```python
from build123d import *

# Parameters (mm, degrees)
SKETCH_1_W          = 48.45
SKETCH_1_H          = 34.2
SKETCH_1_W_2        = 28.45
SKETCH_1_H_2        = 14.2
EXTRUDE_1_DEPTH     = 12.25
SKETCH_2_R          = 1.91
CUT_EXTRUDE_1_DEPTH = 33.083066016
SKETCH_4_W          = 13
SKETCH_4_H          = 13.91
EXTRUDE_1_2_DEPTH   = 74.82
SKETCH_5_W          = 13.91
SKETCH_5_H          = 16.23
EXTRUDE_2_DEPTH     = 16
SKETCH_7_R          = 25.25
SKETCH_7_R_2        = 15.25
EXTRUDE_2_2_DEPTH   = 16.23
SKETCH_15_R         = 1.91
CUT_EXTRUDE_6_DEPTH = 97.964478439
SKETCH_16_W         = 13.91
SKETCH_16_H         = 16.23
EXTRUDE_4_DEPTH     = 10
SKETCH_17_R         = 1.91
CUT_EXTRUDE_7_DEPTH = 102.16913771
SKETCH_18_W         = 48.429544624
SKETCH_18_H         = 6.125
CUT_EXTRUDE_8_DEPTH = 105.840616652
SKETCH_19_W         = 34.2
SKETCH_19_H         = 6.125
CUT_EXTRUDE_9_DEPTH = 10


with BuildPart() as part:
    # 草圖1 → Extrude 1 (new body)
    with BuildSketch(Plane(origin=(0, 0, 0), x_dir=(1, 0, 0), z_dir=(0, 1, 0))):
        Rectangle(SKETCH_1_W, SKETCH_1_H)
        Rectangle(SKETCH_1_W_2, SKETCH_1_H_2, mode=Mode.SUBTRACT)
    extrude(amount=EXTRUDE_1_DEPTH)

    # 草圖2 → 除料-伸長1 (cut, through all)
    with BuildSketch(Plane(origin=(0, 12.25, 0), x_dir=(1, 0, 0), z_dir=(0, 1, 0))):
        with Locations(Location((-19.225, 0, 0), (0, 0, 270))):
            Circle(SKETCH_2_R)
        with Locations(Location((19.225, 0, 0), (0, 0, 270))):
            Circle(SKETCH_2_R)
    extrude(amount=-CUT_EXTRUDE_1_DEPTH, mode=Mode.SUBTRACT)

    # 草圖4 → Extrude 1 2 (add)
    with BuildSketch(Plane.XZ):
        with Locations((17.725, 0)):
            Rectangle(SKETCH_4_W, SKETCH_4_H)
    extrude(amount=EXTRUDE_1_2_DEPTH)

    # 草圖5 → Extrude 2 (add)
    with BuildSketch(Plane.ZY.offset(-11.225)):
        with Locations((0, -66.705)):
            Rectangle(SKETCH_5_W, SKETCH_5_H)
    extrude(amount=EXTRUDE_2_DEPTH)

    # 草圖7 → Extrude 2 2 (add)
    with BuildSketch(Plane(origin=(3.626674765, -74.82, 0), x_dir=(1, 0, 0), z_dir=(0, -1, 0))):
        with Locations((-30.978154344, 0)):
            Circle(SKETCH_7_R)
        with Locations((-30.978154344, 0)):
            Circle(SKETCH_7_R_2, mode=Mode.SUBTRACT)
    extrude(amount=-EXTRUDE_2_2_DEPTH)

    # 草圖15 → 除料-伸長6 (cut, through all)
    with BuildSketch(Plane(origin=(0, 0, -6.955), x_dir=(-1, 0, 0), z_dir=(0, 0, -1))):
        with Locations((-4.073383248, -66.705)):
            Circle(SKETCH_15_R)
    extrude(amount=-CUT_EXTRUDE_6_DEPTH, mode=Mode.SUBTRACT)

    # 草圖16 → 填料-伸長4 (add)
    with BuildSketch(Plane(origin=(-60, 0, 0), x_dir=(0, 0, -1), z_dir=(1, 0, 0))):
        with Locations((0, -66.705)):
            Rectangle(SKETCH_16_W, SKETCH_16_H)
    extrude(amount=EXTRUDE_4_DEPTH)

    # 草圖17 → 除料-伸長7 (cut, through all)
    with BuildSketch(Plane(origin=(0, 0, -6.955), x_dir=(-1, 0, 0), z_dir=(0, 0, -1))):
        with Locations((55.812362827, -66.705)):
            Circle(SKETCH_17_R)
    extrude(amount=-CUT_EXTRUDE_7_DEPTH, mode=Mode.SUBTRACT)

    # 草圖18 → 除料-伸長8 (cut, through all)
    with BuildSketch(Plane(origin=(0, 0, -17.1), x_dir=(-1, 0, 0), z_dir=(0, 0, -1))):
        with Locations((0.010227688, 9.1875)):
            Rectangle(SKETCH_18_W, SKETCH_18_H)
    extrude(amount=-CUT_EXTRUDE_8_DEPTH, mode=Mode.SUBTRACT)

    # 草圖19 → 除料-伸長9 (cut)
    with BuildSketch(Plane.ZY.offset(-24.204544624)):
        with Locations((0, 9.1875)):
            Rectangle(SKETCH_19_W, SKETCH_19_H)
    extrude(amount=-CUT_EXTRUDE_9_DEPTH, mode=Mode.SUBTRACT)


solid = part.part
```
Read the model definition and answer for the solid it produces. Units are mm, in the model's axes. A direction names the side the tool comes from. Give positions to 0.01 mm unless a question says otherwise; leave off trailing zeros. Write each loop counter-clockwise with the first axis right and the second up, starting at its lowest first coordinate (ties: lowest second). Pieces come first, ordered by that corner, then holes. Notation, with made-up numbers: (45, -30) -> (69, -30) arc R20 ccw to (69, 7) -> close; hole circle Ø2 at (64, -31.75). An arc over 180 degrees is marked (long way). Answer as a JSON object with one key per item and string values.
1) Section B-B on y = -61.5 is taken. Write down the section's boundary in (x, z) (3 decimals).
Findings below:
{"outline": "(-60, -6.955) -> (-51.625, -6.955) arc R25.25 ccw to (-3.078, -6.955) -> (24.225, -6.955) -> (24.225, 6.955) -> (-3.078, 6.955) arc R25.25 ccw to (-51.625, 6.955) -> (-60, 6.955) -> close; hole circle Ø30.5 at (-27.351, 0)"}
2) Straight lines are drawn through the part: probe 1 along X at (y, z) = (2, 0) (3 decimals); probe 2 along Y at (x, z) = (-13, 12) (3 decimals); probe 3 along Z at (x, y) = (-26.5, -60). For each, find the intervals that lie inside material, in ascending order. Write a range as from..to.
Findings below:
{"probe 1": "x = -24.225..-21.135, -17.315..-14.225, 14.225..17.315, 21.135..24.225", "probe 2": "y = -74.82..-58.59, 0..6.125", "probe 3": "z = -25.24..-15.23, 15.23..25.24"}
3) Section A-A on z = 0 is taken. Write down the section's boundary in (x, y) (3 decimals).
Findings below:
{"outline": "(-60, -74.82) -> (-42.601, -74.82) -> (-42.601, -58.59) -> (-60, -58.59) -> close; (-24.225, 0) -> (-21.135, 0) -> (-21.135, 6.125) -> (-24.225, 6.125) -> close; (-17.315, 0) -> (-14.225, 0) -> (-14.225, 6.125) -> (-17.315, 6.125) -> close; (-12.101, -74.82) -> (24.225, -74.82) -> (24.225, 6.125) -> (21.135, 6.125) -> (21.135, 0) -> (17.315, 0) -> (17.315, 6.125) -> (14.225, 6.125) -> (14.225, 0) -> (11.225, 0) -> (11.225, -58.59) -> (-12.101, -58.59) -> close; hole circle Ø3.82 at (-55.812, -66.705); hole circle Ø3.82 at (4.073, -66.705)"}
4) Flat-ended cylindrical pins translate along their axes: pin 1 Ø3.5 at (x, y) = (-55.81, -66.7) entering from -Z; pin 2 Ø1.8 at (x, y) = (-12, 3.5) entering from +Z; pin 3 Ø3 at (x, y) = (10.5, -53) entering from -Z (3 decimals); pin 4 Ø3 at (y, z) = (-64.5, -17) entering from +X. Find the tip coordinate at first contact, or state that the pin passes through.
Findings below:
{"pin 1": "passes through", "pin 2": "stops at z = 17.1", "pin 3": "stops at z = -6.955", "pin 4": "stops at x = -7.42"}
5) Section C-C on x = -34 is taken. Write down the section's boundary in (y, z), then the cut area to 3 significant figures.
Findings below:
{"outline": "(-74.82, -24.36) -> (-58.59, -24.36) -> (-58.59, -13.72) -> (-74.82, -13.72) -> close; (-74.82, 13.72) -> (-58.59, 13.72) -> (-58.59, 24.36) -> (-74.82, 24.36) -> close", "area": "345 mm^2"}
6) A tool of negligible diameter and unlimited length cuts with its end or side. For faces 5 (the flat face through (-56, -69, -6.955)), 6 (the flat face through (17, -46, 6.955)), 7 (the flat face through (19, 0, 0)), from which of +Z, -Z, +X, -X, +Y, -Y can it reach the whole face along a straight path? Write none if from no direction.
Findings below:
{"face 5": "-Z, -X, +Y, -Y", "face 6": "+Z, +X, -Y", "face 7": "+Y"}
7) Section D-D on x = 3.5 is taken. Write down the section's boundary in (y, z) (3 decimals), then the cut area to 3 significant figures.
Findings below:
{"outline": "(-74.82, -6.955) -> (-68.527, -6.955) -> (-68.527, 6.955) -> (-74.82, 6.955) -> close; (-64.883, -6.955) -> (-58.59, -6.955) -> (-58.59, 6.955) -> (-64.883, 6.955) -> close; (0, -17.1) -> (6.125, -17.1) -> (6.125, -7.1) -> (0, -7.1) -> close; (0, 7.1) -> (6.125, 7.1) -> (6.125, 17.1) -> (0, 17.1) -> close", "area": "298 mm^2"}
8) For a pull along Z with two mould halves and no side action, classify faces 1 (the cylindrical face through (-27.808, -66.819, -25.246)), 2 (the flat face through (24.225, -25, 0)), 3 (the cylindrical face through (-26.895, -66.819, 25.246)), 4 (the cylindrical face through (17.36, 3.11, -0.41)) as pulls with the +Z half, pulls with the -Z half, needs draft (parallel to the pull), parting line crosses it, or undercut.
Findings below:
{"face 1": "pulls with the -Z half", "face 2": "needs draft", "face 3": "pulls with the +Z half", "face 4": "undercut"}
